```python
from build123d import *

# Parameters (mm, degrees)
SKETCH1_W                   = 25.4
SKETCH1_H                   = 25.4
SKETCH1_W_2                 = 19.05
SKETCH1_H_2                 = 19.05
BOSS_EXTRUDE1_DEPTH         = 177.8
F_21_0_159_DIAMETER_HOLE1_D = 4.0386
LPATTERN1_COUNT             = 13
LPATTERN1_PITCH             = 12.7
F_21_0_159_DIAMETER_HOLE2_D = 4.0386
LPATTERN2_COUNT             = 13
LPATTERN2_PITCH             = 12.7


with BuildPart() as part:
    # Sketch1 → Boss-Extrude1 (new body)
    with BuildSketch(Plane(origin=(0, 0, 0), x_dir=(1, 0, 0), z_dir=(0, 1, 0))):
        Rectangle(SKETCH1_W, SKETCH1_H)
        Rectangle(SKETCH1_W_2, SKETCH1_H_2, mode=Mode.SUBTRACT)
    extrude(amount=BOSS_EXTRUDE1_DEPTH)

    # #21 (0.159) Diameter Hole1 (through all)
    with Locations(Plane.ZY.offset(12.7)):
        with Locations((0, 12.7)):
            f_21_0_159_diameter_hole1 = Hole(F_21_0_159_DIAMETER_HOLE1_D / 2)

    # LPattern1: #21 (0.159) Diameter Hole1 ×13
    with Locations(*[(0, i * LPATTERN1_PITCH, 0) for i in range(1, LPATTERN1_COUNT)]):
        add(f_21_0_159_diameter_hole1, mode=Mode.SUBTRACT)

    # #21 (0.159) Diameter Hole2 (through all)
    with Locations(Plane(origin=(0, 0, -12.7), x_dir=(-1, 0, 0), z_dir=(0, 0, -1))):
        with Locations((0, 12.7)):
            f_21_0_159_diameter_hole2 = Hole(F_21_0_159_DIAMETER_HOLE2_D / 2)

    # LPattern2: #21 (0.159) Diameter Hole2 ×13
    with Locations(*[(0, i * LPATTERN2_PITCH, 0) for i in range(1, LPATTERN2_COUNT)]):
        add(f_21_0_159_diameter_hole2, mode=Mode.SUBTRACT)


solid = part.part
```
For this review, take the finished solid that the model builds, in its own axes (mm). A direction names the side the tool comes from. Round coordinates to 2 decimals unless told otherwise and drop trailing zeros. Write each loop counter-clockwise with the first axis right and the second up, starting at its lowest first coordinate (ties: lowest second). Pieces come first, ordered by that corner, then holes.
1) Take a section at C-C on y = 30. Give the boundary of the cut face in (x, z) (3 decimals).
Answer below:
outline: (-12.7, -12.7) - (12.7, -12.7) - (12.7, 12.7) - (-12.7, 12.7) - close; hole (-9.525, -9.525) - (9.525, -9.525) - (9.525, 9.525) - (-9.525, 9.525) - close
2) Machinability: for faces 1 (the face through (-2, 88, 9.525)), 2 (the face through (-0.44, 112.33, -11.09)), which of the approach directions +Z, -Z, +X, -X, +Y, -Y give a long, thin tool a straight path to every point of the face, cutting with its end or side? Answer none if there is none.
Answer below:
face 1: +Y, -Y
face 2: +Z, -Z
3) Take a section at B-B on x = 11. State how many separate pieces and enclosed holes the cut face has, then the cut area to 3 significant figures.
Answer below:
separate pieces: 1
enclosed holes: 13
area: 4,350 mm2
4) For line 1 along Z through (x, y) = (-10.55, 88.9); line 2 along X through (y, z) = (30.5, -4.25) (3 decimals), list the stretches that pass through material, from the lowest coordinate up.
Answer below:
line 1: z = -12.7 to -2.02, 2.02 to 12.7
line 2: x = -12.7 to -9.525, 9.525 to 12.7
5) Take a section at A-A on y = 114.3. Give the boundary of the cut face in (x, z) (3 decimals), then the cut area to 3 significant figures.
Answer below:
outline: (-12.7, -12.7) - (-2.019, -12.7) - (-2.019, -9.525) - (-9.525, -9.525) - (-9.525, -2.019) - (-12.7, -2.019) - close; (-12.7, 2.019) - (-9.525, 2.019) - (-9.525, 9.525) - (-2.019, 9.525) - (-2.019, 12.7) - (-12.7, 12.7) - close; (2.019, -12.7) - (12.7, -12.7) - (12.7, -2.019) - (9.525, -2.019) - (9.525, -9.525) - (2.019, -9.525) - close; (2.019, 9.525) - (9.525, 9.525) - (9.525, 2.019) - (12.7, 2.019) - (12.7, 12.7) - (2.019, 12.7) - close
area: 231 mm2
6) Mouldability with a two-part tool opening along Z and no side actions: class faces 3 (the face through (3, 88, -12.7)), 4 (the face through (11.13, 112.33, 0.44)), 5 (the face through (-11.09, 52.802, 0.263)), 6 (the face through (-0.263, 65.502, -11.09)) as +Z half, -Z half, draft (parallel to the pull), parting line (faces both ways), or undercut.
Answer below:
face 3: -Z half
face 4: undercut
face 5: undercut
face 6: draft
7) Take a section at D-D on z = -5.75. Give the boundary of the cut face in (x, y) (3 decimals).
Answer below:
outline: (-12.7, 0) - (-9.525, 0) - (-9.525, 177.8) - (-12.7, 177.8) - close; (9.525, 0) - (12.7, 0) - (12.7, 177.8) - (9.525, 177.8) - close
